Input: part model. Units: mm. Frame: model coordinates. Face numbers are marked on the shaded views. A direction names the side the tool comes from. Coordinates: 2 decimals unless noted, no trailing zeros. Loops run counter-clockwise (first coordinate to the right, second up) from the corner with the lowest first, then second, coordinate; pieces in that order, holes last.
Item 1: Section C-C on z = -53. Return loops of the section in (x, y).
Item 2: Reachability of the marked faces 1 and 2 from +Z, -Z, +X, -X, +Y, -Y: full face, straight path, thin tool, end or side. Return the list, or none.
Item 3: Ray query, line 1 along Z through (x, y) = (29.5, 100.5); line 2 along Z through (x, y) = (7, 38); line 3 along Y through (x, z) = (22.5, -118). Return the intervals inside material, ascending.
Item 4: Section B-B on x = 24. Return loops of the section in (y, z), and give its area (3 significant figures).
Item 5: Contact query for flat-ended pins moving along their axis: P1, Ø21, axis at x = 29, z = -48.5, coming from the +Y side; P2, Ø1.5, axis at x = 13.5, y = 82, coming from the -Z side; P3, Ø1, axis at x = 10.5, y = 112, coming from the -Z side. Output: stop coordinate, or through.
Item 6: Pull-direction query (Y, two-part tool) for the marked faces 3, 4 and 5; classes: released by +Y, released by -Y, zero draft, split by the parting line, or undercut.
Item 7: Section A-A on y = 104.5. Return loops of the section in (x, z).
```python
from build123d import *

# Parameters (mm, degrees)
EXTRUDE_1_DEPTH     = 3
EXTRUDE_2_DEPTH     = 38.5
CUT_EXTRUDE_5_DEPTH = 3


with BuildPart() as part:
    # 草图1 → 凸台-拉伸1 (new body)
    with BuildSketch(Plane(origin=(0, 0, 0), x_dir=(0, 0, -1), z_dir=(1, 0, 0))):
        with BuildLine():
            Line((-132.35662508, 0), (146.100403215, 0))
            ThreePointArc((146.100403215, 0), (157.691079906, 3.488397737), (165.431005137, 12.794646302))
            Line((165.431005137, 12.794646302), (197.861688802, 89.196549138))
            ThreePointArc((197.861688802, 89.196549138), (196.566084988, 108.16010172), (180.495077268, 118.30986165))
            Line((180.495077268, 118.30986165), (-272.113220038, 160.825649707))
            ThreePointArc((-272.113220038, 160.825649707), (-293.452890241, 148.016026014), (-287.575750229, 123.830757588))
            Line((-287.575750229, 123.830757588), (-145.855164884, 4.913066695))
            ThreePointArc((-145.855164884, 4.913066695), (-139.53904809, 1.266454963), (-132.35662508, 0))
        make_face()
    extrude(amount=EXTRUDE_1_DEPTH)

    # 草图2 → 凸台-拉伸2 (add)
    with BuildSketch(Plane(origin=(3, 0, 0), x_dir=(0, 0, -1), z_dir=(1, 0, 0))):
        with BuildLine():
            Line((-272.113220038, 160.825649707), (180.495077268, 118.30986165))
            ThreePointArc((180.495077268, 118.30986165), (196.566084988, 108.16010172), (197.861688802, 89.196549138))
            Line((197.861688802, 89.196549138), (165.431005137, 12.794646302))
            ThreePointArc((165.431005137, 12.794646302), (157.691079906, 3.488397737), (146.100403215, 0))
            Line((146.100403215, 0), (-132.35662508, 0))
            ThreePointArc((-132.35662508, 0), (-139.53904809, 1.266454963), (-145.855164884, 4.913066695))
            Line((-145.855164884, 4.913066695), (-287.575750229, 123.830757588))
            ThreePointArc((-287.575750229, 123.830757588), (-293.452890241, 148.016026014), (-272.113220038, 160.825649707))
        make_face()
        with BuildLine():
            Line((-272.487313445, 156.843181362), (180.120983861, 114.327393305))
            ThreePointArc((180.120983861, 114.327393305), (193.130847253, 106.110920981), (194.179669388, 90.759473652))
            Line((194.179669388, 90.759473652), (161.748985724, 14.357570816))
            ThreePointArc((161.748985724, 14.357570816), (155.483331965, 6.823941025), (146.100403215, 4))
            Line((146.100403215, 4), (-132.35662508, 4))
            ThreePointArc((-132.35662508, 4), (-138.170967517, 5.025225447), (-143.284014445, 7.977244467))
            Line((-143.284014445, 7.977244467), (-285.004599791, 126.894935361))
            ThreePointArc((-285.004599791, 126.894935361), (-289.762284562, 146.473485991), (-272.487313445, 156.843181362))
        make_face(mode=Mode.SUBTRACT)
    extrude(amount=EXTRUDE_2_DEPTH)

    # 草图4 → 切除-拉伸5 (cut)
    with BuildSketch(Plane(origin=(3, 0, 0), x_dir=(0, 0, -1), z_dir=(1, 0, 0))):
        with BuildLine():
            Line((-272.487313445, 156.843181362), (180.120983861, 114.327393305))
            ThreePointArc((180.120983861, 114.327393305), (193.130847253, 106.110920981), (194.179669388, 90.759473652))
            Line((194.179669388, 90.759473652), (161.748985724, 14.357570816))
            ThreePointArc((161.748985724, 14.357570816), (155.483331965, 6.823941025), (146.100403215, 4))
            Line((146.100403215, 4), (-132.35662508, 4))
            ThreePointArc((-132.35662508, 4), (-138.170967517, 5.025225447), (-143.284014445, 7.977244467))
            Line((-143.284014445, 7.977244467), (-285.004599791, 126.894935361))
            ThreePointArc((-285.004599791, 126.894935361), (-289.762284562, 146.473485991), (-272.487313445, 156.843181362))
        make_face()
    extrude(amount=-CUT_EXTRUDE_5_DEPTH, mode=Mode.SUBTRACT)


solid = part.part
```
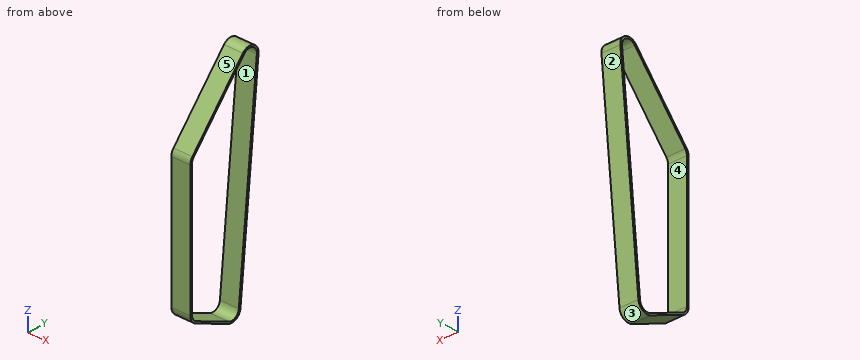
Results found:
1. outline: (0, 0) - (41.5, 0) - (41.5, 4) - (0, 4) - close; (0, 126.27) - (41.5, 126.27) - (41.5, 130.29) - (0, 130.29) - close
2. face 1: +X, -X
2. face 2: -Z, +X, -X, +Y
3. line 1: z = -199.3 to -195.25, 253.55 to 259.77
3. line 2: z = -176.13 to -171.78, 179.06 to 185.29
3. line 3: y = 0 to 4, 120.16 to 124.18
4. outline: (0, -146.1) arc R21 ccw to (12.79, -165.43) - (89.2, -197.86) arc R21 ccw to (118.31, -180.5) - (160.83, 272.11) arc R21 ccw to (123.83, 287.58) - (4.91, 145.86) arc R21 ccw to (0, 132.36) - close; hole (4, -146.1) arc R17 ccw to (14.36, -161.75) - (90.76, -194.18) arc R17 ccw to (114.33, -180.12) - (156.84, 272.49) arc R17 ccw to (126.89, 285) - (7.98, 143.28) arc R17 ccw to (4, 132.36) - close
4. area: 4,480 mm2
5. P1: stops at y = 131.7
5. P2: stops at z = -195.13
5. P3: stops at z = -194.1
6. face 3: split by the parting line
6. face 4: undercut
6. face 5: released by -Y
7. outline: (0, -198.3) - (41.5, -198.3) - (41.5, -193.98) - (0, -193.98) - close; (0, 258.32) - (41.5, 258.32) - (41.5, 264.54) - (0, 264.54) - close
